Verification items for this drawing (mm, ordinates from the low corner). Give positions to 0.01 mm unless a question says otherwise; leave off trailing zeros. Loops run counter-clockwise (first coordinate to the right, second up) from the corner with the lowest first, then second, coordinate; pieces in that order, holes last. Notation, with made-up numbers: M 4,5.25 L 17,5.25 A23 cw 17,26.25 Z; hole C -10.5,23 d2. An arc over 180 degrees is marked long. Answer in a Markdown table with one row per item.
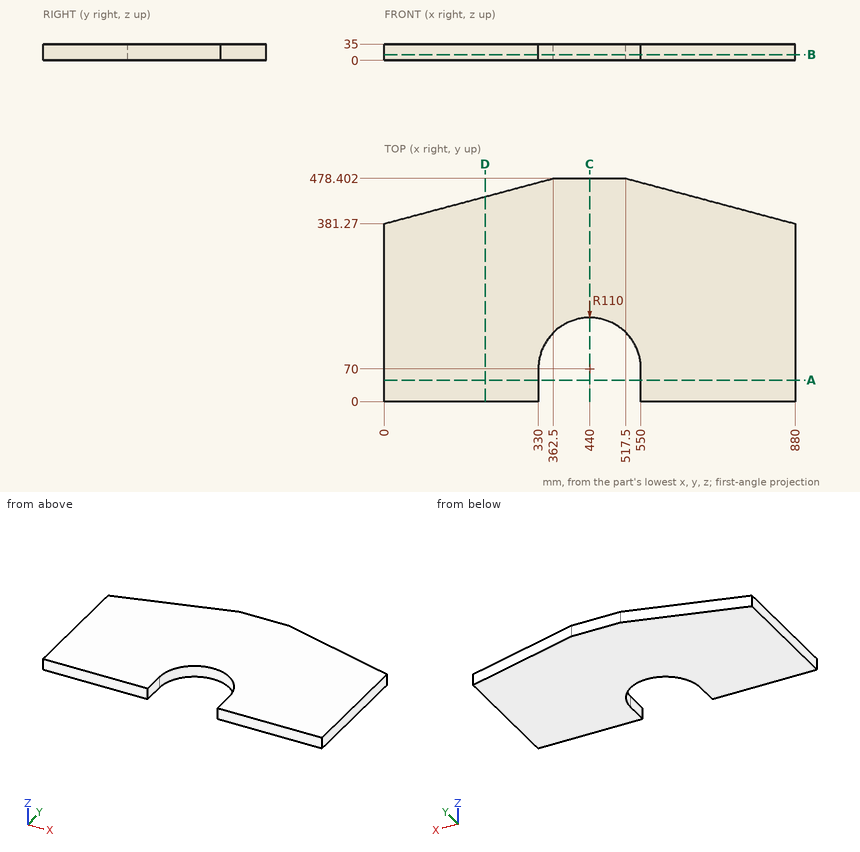
Item 1: Sectioned sample at B-B (z = 12). Record the cut outline in (x, y), and give its area (3 significant figures).
Reported:
| item | result |
|---|---|
| outline | M 0,0 L 330,0 L 330,70 A110 cw 550,70 L 550,0 L 880,0 L 880,381.27 L 517.5,478.4 L 362.5,478.4 L 0,381.27 Z |
| area | 351,000 mm^2 |
Item 2: Sectioned sample at D-D (x = 216). Record the cut outline in (y, z).
Reported:
| item | result |
|---|---|
| outline | M 0,0 L 439.15,0 L 439.15,35 L 0,35 Z |
Item 3: Go/stop test with flat-tipped pins: pin 1 (2 mm diameter, centred on x = 468.5, z = 10.5, fed in from -Y); pin 2 (1.5 mm diameter, centred on x = 625, z = 4, fed in from +Y). Record where each tip stops, or that it passes through.
Reported:
| item | result |
|---|---|
| pin 1 | stops at y = 175.97 |
| pin 2 | stops at y = 449.8 |
Item 4: Sectioned sample at C-C (x = 440). Record the cut outline in (y, z).
Reported:
| item | result |
|---|---|
| outline | M 180,0 L 478.4,0 L 478.4,35 L 180,35 Z |
Item 5: Sectioned sample at A-A (y = 46). Record the cut outline in (x, z), and give its area (3 significant figures).
Reported:
| item | result |
|---|---|
| outline | M 0,0 L 330,0 L 330,35 L 0,35 Z; M 550,0 L 880,0 L 880,35 L 550,35 Z |
| area | 23,100 mm^2 |
Item 6: Scan lines: L1, parallel to X at y = 36.5, z = 25; L2, parallel to X at y = 144, z = 15; L3, parallel to Y at x = 414, z = 14. Record each from-to range of solid material in increasing order. Write a range as [from, to].
Reported:
| item | result |
|---|---|
| L1 | x = [0, 330], [550, 880] |
| L2 | x = [0, 358.61], [521.39, 880] |
| L3 | y = [176.88, 478.4] |
